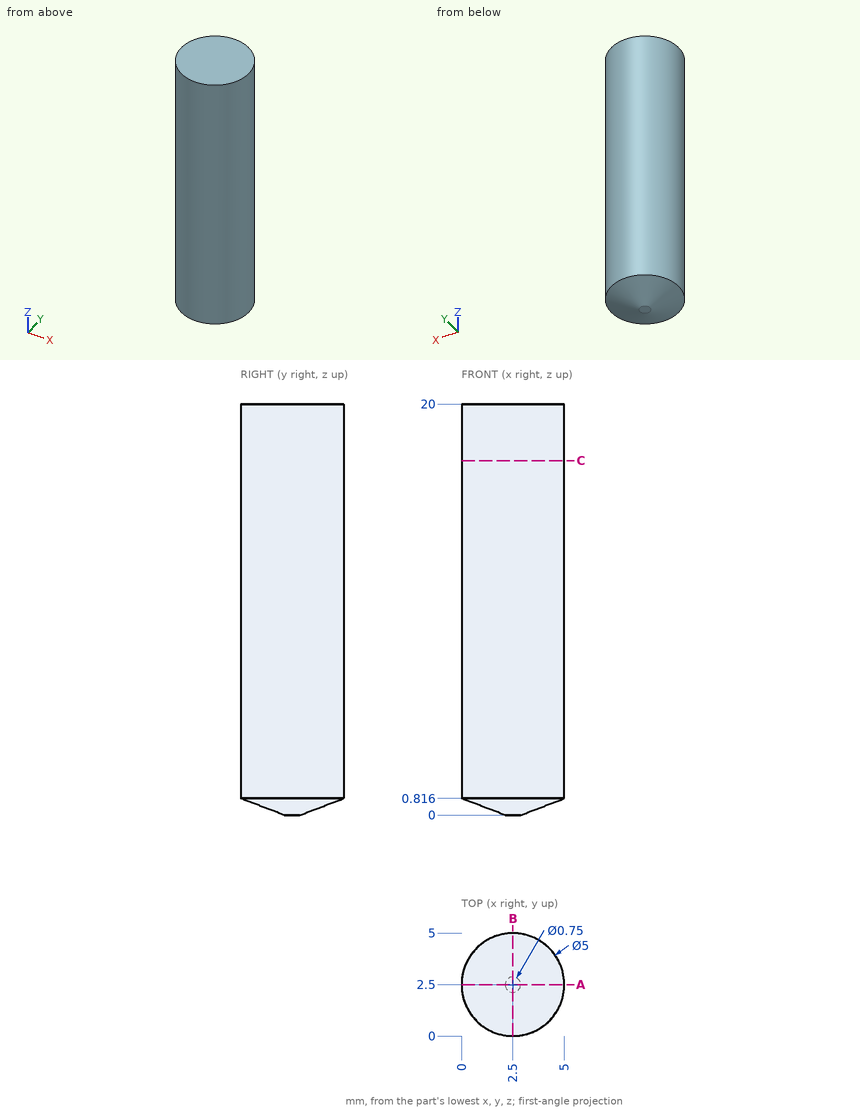
Here's the drawing with two shaded views (mm, measured from the low corner). I have some questions. Coordinates: 2 decimals unless noted, no trailing zeros. Loops run counter-clockwise (first coordinate to the right, second up) from the corner with the lowest first, then second, coordinate; pieces in that order, holes last. Notation, with made-up numbers: M -10.75,-29.75 L 28.25,-29.75 A23 ccw 28.25,2.25 Z; hole C 37.25,87 d5. An arc over 180 degrees is marked long. Return JSON: item names as keys, results as strings. Group by question number.
Item 1: Imagine slicing it at C-C (z = 17.25). Please give me the cut outline in (x, y), and give its area (3 significant figures).
Item 2: Imagine slicing it at A-A (y = 2.5). Please give me the cut outline in (x, z) (1 decimal).
Item 3: I'm going to push a flat-ended pin straight in: pin 1 Ø1.5 at (x, y) = (1, 1) entering from -Z. Where does the tip first touch, or does it pass through?
Item 4: If I drill on L1, parallel to X at y = 2.6, z = 3; L2, parallel to Y at x = 2.8, z = 9.5; L3, parallel to Z at x = 1.95, y = 1.1, over which ranges is the centre line in solid material (lowest first)? Write a range as from..to.
Verdict:
{
 "1": {"outline": "C 2.5,2.5 d5", "area": "19.6 mm^2"},
 "2": {"outline": "M 0,0.8 L 2.1,0 L 2.9,0 L 5,0.8 L 5,20 L 0,20 Z"},
 "3": {"pin 1": "stops at z = 0.38"},
 "4": {"L1": "x = 0..5", "L2": "y = 0.02..4.98", "L3": "z = 0.43..20"}
}
